For this review, take the finished solid that the model builds, in its own axes (mm). Face numbers are marked on the shaded views. A direction names the side the tool comes from. Coordinates: 2 decimals unless noted, no trailing zeros. Loops run counter-clockwise (first coordinate to the right, second up) from the corner with the lowest first, then second, coordinate; pieces in that order, holes last. Notation, with made-up numbers: (71.25, 8) - (108.25, 8) arc R34 ccw to (108.25, 40) - close; hole circle Ø11 at (66.5, 82.25). An arc over 180 degrees is marked (long way). One line per item, written item: value. Start each with the question number.
1. Take a section at A-A, the plane z = 6. State the section outline as (x, y) points, and give its area (3 significant figures).
2. Insertion check: pin 1 (2.5 mm diameter, centred on x = 21, y = -23, fed in from +Z); pin 2 (8 mm diameter, centred on x = 8.5, z = 46.5, fed in from +Y); pin 3 (8 mm diameter, centred on y = -3.5, z = 59, fed in from +X); pin 4 (6 mm diameter, centred on x = 18.5, z = 77.5, fed in from -Y). Each pin has a flat end and moves straight along its axis. Give the tip position at first contact, or say it passes through.
3. To check wall thickness, follow line 1 (X direction, y = 0, z = 55); line 2 (Y direction, x = -16.5, z = 53.5); line 3 (Y direction, x = -17, z = 64.5). State the ranges of each line that lie inside material, in increasing order. Write a range as from..to.
4. The part is to be moulded in two halves that separate along Y. For the marked faces 3 and 4, say which applies: released by +Y, released by -Y, zero draft, split by the parting line, or undercut.
5. For the marked faces 1 and 2, list the 3-axis set-ups (+Z, -Z, +X, -X, +Y, -Y) from which the entire face can be reached by the end or side of a thin tool; tool diameter is ignored.
6. Take a section at C-C, the plane z = 21.5. State the section outline as (x, y) points.
7. Take a section at B-B, the plane x = 28.5. State the section outline as (y, z) points.
8. Take a section at D-D, the plane y = 0. Count the separate pieces of the cut face and the enclosed holes in it, and give its area (3 significant figures).
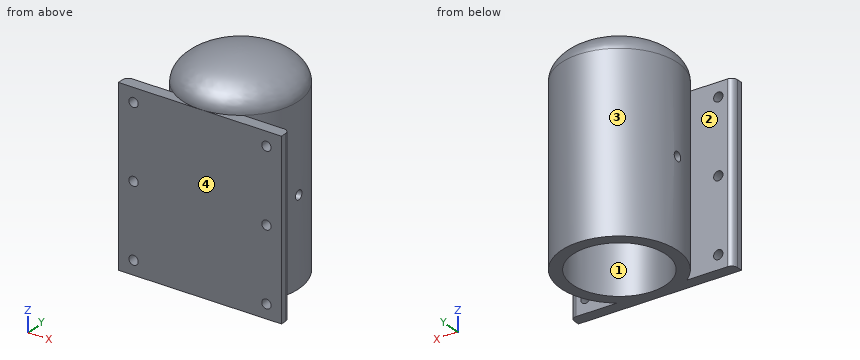
```python
from build123d import *

# Parameters (mm, degrees)
SKETCH1_R               = 20
BOSS_EXTRUDE1_DEPTH     = 75
CUT_EXTRUDE2_DEPTH      = 87.458082329
CUT_EXTRUDE2_DEPTH_BACK = 87.458082329
SKETCH3_R               = 2
SKETCH2_R               = 2
CUT_EXTRUDE3_DEPTH      = 10
SKETCH2_4_R             = 2
CUT_EXTRUDE4_DEPTH      = 10


with BuildPart() as part:
    # Sketch1 → Boss-Extrude1 (new body)
    with BuildSketch(Plane.XY):
        with BuildLine():
            Line((-32.5, -20), (-15, -20))
            ThreePointArc((-15, -20), (0, 25), (15, -20))
            Line((15, -20), (32.5, -20))
            ThreePointArc((32.5, -20), (34.267766953, -20.732233047), (35, -22.5))
            Line((35, -22.5), (35, -25))
            Line((35, -25), (-35, -25))
            Line((-35, -25), (-35, -22.5))
            ThreePointArc((-35, -22.5), (-34.267766953, -20.732233047), (-32.5, -20))
        make_face()
        Circle(SKETCH1_R, mode=Mode.SUBTRACT)
    extrude(amount=BOSS_EXTRUDE1_DEPTH)

    # Sketch3 → Cut-Extrude2 (cut, two sides: drawn at the far end of the back side and taken through both)
    with BuildSketch(Plane(origin=(0, 0, 0), x_dir=(0, 0, -1), z_dir=(1, 0, 0)).offset(-CUT_EXTRUDE2_DEPTH_BACK)):
        with Locations((-37.5, 0)):
            Circle(SKETCH3_R)
    extrude(amount=CUT_EXTRUDE2_DEPTH + CUT_EXTRUDE2_DEPTH_BACK, mode=Mode.SUBTRACT)

    # Sketch4 → Revolve1 (revolve)
    with BuildSketch(Plane(origin=(0, 0, 0), x_dir=(0, 0, -1), z_dir=(1, 0, 0)), mode=Mode.PRIVATE) as revolve1_sk:
        with BuildLine():
            Line((-87.5, 0), (-84.5, 0))
            add(Edge.make_bspline(
                [(-75, 22), (-75.216185099, 22), (-75.636923923, 21.95894914), (-76.546271577, 21.69469962), (-77.844229013, 20.93469698), (-79.554525777, 19.135071068), (-81.193703824, 16.461120363), (-82.603978079, 13.036619939), (-83.678181323, 9.024220506), (-84.34830956, 4.618558705), (-84.5, 1.528633227), (-84.5, 0)],
                knots=[0, 0, 0, 0, 0.09817477, 0.196349541, 0.392699082, 0.589048623, 0.785398163, 0.981747704, 1.178097245, 1.374446786, 1.570796327, 1.570796327, 1.570796327, 1.570796327], degree=3))
            Line((-75, 22), (-75, 25))
            add(Edge.make_bspline(
                [(-75, 25), (-87.5, 25), (-87.5, 0)],
                knots=[0, 0, 0, 1.570796327, 1.570796327, 1.570796327], degree=2, weights=[1, 0.707106781, 1]))
        make_face()
    revolve(revolve1_sk.sketch.rotate(Axis((0, 0, 87.5), (0, 0, -1)), 90), axis=Axis((0, 0, 87.5), (0, 0, -1)))

    # Sketch2 → Cut-Extrude3 (cut)
    with BuildSketch(Plane(origin=(0, -20, 0), x_dir=(1, 0, 0), z_dir=(0, 1, 0))):
        with Locations(Location((28.5, -69, 0), (0, 0, 180))):
            Circle(SKETCH2_R)
    extrude(amount=-CUT_EXTRUDE3_DEPTH, mode=Mode.SUBTRACT)

    # Sketch2_4 → Cut-Extrude4 (cut)
    with BuildSketch(Plane(origin=(0, -20, 0), x_dir=(1, 0, 0), z_dir=(0, 1, 0))):
        with Locations(Location((-28.5, -37.5, 0), (0, 0, 180))):
            Circle(SKETCH2_4_R)
        with Locations(Location((-28.5, -6, 0), (0, 0, 180))):
            Circle(SKETCH2_4_R)
        with Locations(Location((-28.5, -69, 0), (0, 0, 270))):
            Circle(SKETCH2_4_R)
        with Locations(Location((28.5, -6, 0), (0, 0, 270))):
            Circle(SKETCH2_4_R)
        with Locations(Location((28.5, -37.5, 0), (0, 0, 180))):
            Circle(SKETCH2_4_R)
    extrude(amount=-CUT_EXTRUDE4_DEPTH, mode=Mode.SUBTRACT)


solid = part.part
```
Solutions:
1. outline: (-35, -25) - (-30.5, -25) - (-30.5, -20) - (-32.5, -20) arc R2.5 ccw to (-35, -22.5) - close; (-26.5, -25) - (26.5, -25) - (26.5, -20) - (15, -20) arc R25 ccw (long way) to (-15, -20) - (-26.5, -20) - close; (30.5, -25) - (35, -25) - (35, -22.5) arc R2.5 ccw to (32.5, -20) - (30.5, -20) - close; hole circle Ø40 at (0, 0)
1. area: 912 mm2
2. pin 1: z = 75
2. pin 2: y = 24.59
2. pin 3: x = 25
2. pin 4: y = -25
3. line 1: -25..-20, 20..25
3. line 2: -25..-20, -18.78..-11.3, 11.3..18.78
3. line 3: -25..-20, -18.33..-10.54, 10.54..18.33
4. face 3: undercut
4. face 4: released by -Y
5. face 1: -Z
5. face 2: +Z, -Z, -X
6. outline: (-35, -25) - (35, -25) - (35, -22.5) arc R2.5 ccw to (32.5, -20) - (15, -20) arc R25 ccw (long way) to (-15, -20) - (-32.5, -20) arc R2.5 ccw to (-35, -22.5) - close; hole circle Ø40 at (0, 0)
7. outline: (-25, 0) - (-20, 0) - (-20, 4) - (-25, 4) - close; (-25, 8) - (-20, 8) - (-20, 35.5) - (-25, 35.5) - close; (-25, 39.5) - (-20, 39.5) - (-20, 67) - (-25, 67) - close; (-25, 71) - (-20, 71) - (-20, 75) - (-25, 75) - close
8. separate pieces: 3
8. enclosed holes: 0
8. area: 878 mm2
